Can you work these out from the model? Positions are in its coordinate system, mm. Give positions to 0.01 mm unless a question says otherwise; leave off trailing zeros. Order: outer loops, then holes, each group sorted by start corner. A loop starts at its lowest first (then second) coordinate and runs counter-clockwise, first axis right, second up. Notation, with made-up numbers: (7, -2.5) -> (28, -2.5) arc R24 cw to (28, 27.5) -> close; hole circle Ø10 at (28, 48). An arc over 180 degrees is marked (long way). Answer as a JSON object with one key per item and string values.
```python
from build123d import *

# Parameters (mm, degrees)
SKETCH1_R           = 2
SKETCH1_W           = 56
SKETCH1_H           = 56
BOSS_EXTRUDE1_DEPTH = 1
SKETCH3_W           = 56
SKETCH3_H           = 56
BOSS_EXTRUDE3_DEPTH = 1


with BuildPart() as part:
    # Sketch1 → Boss-Extrude1 (new body)
    with BuildSketch(Plane.XY):
        with BuildLine():
            Line((40, -13), (40, 13))
            ThreePointArc((40, 13), (38.828427125, 15.828427125), (36, 17))
            ThreePointArc((36, 17), (33.171572875, 18.171572875), (32, 21))
            Line((32, 21), (32, 32))
            Line((32, 32), (21, 32))
            ThreePointArc((21, 32), (18.171572875, 33.171572875), (17, 36))
            ThreePointArc((17, 36), (15.828427125, 38.828427125), (13, 40))
            Line((13, 40), (-13, 40))
            ThreePointArc((-13, 40), (-15.828427125, 38.828427125), (-17, 36))
            ThreePointArc((-17, 36), (-18.171572875, 33.171572875), (-21, 32))
            Line((-21, 32), (-32, 32))
            Line((-32, 32), (-32, 9))
            ThreePointArc((-32, 9), (-33.464466094, 5.464466094), (-37, 4))
            ThreePointArc((-37, 4), (-41, 0), (-37, -4))
            ThreePointArc((-37, -4), (-33.464466094, -5.464466094), (-32, -9))
            Line((-32, -9), (-32, -32))
            Line((-32, -32), (-9, -32))
            ThreePointArc((-9, -32), (-5.464466094, -33.464466094), (-4, -37))
            ThreePointArc((-4, -37), (0, -41), (4, -37))
            ThreePointArc((4, -37), (5.464466094, -33.464466094), (9, -32))
            Line((9, -32), (32, -32))
            Line((32, -32), (32, -21))
            ThreePointArc((32, -21), (33.171572875, -18.171572875), (36, -17))
            ThreePointArc((36, -17), (38.828427125, -15.828427125), (40, -13))
        make_face()
        with Locations((-37, 0)):
            Circle(SKETCH1_R, mode=Mode.SUBTRACT)
        with Locations((-13, 36)):
            Circle(SKETCH1_R, mode=Mode.SUBTRACT)
        with Locations((0, -37)):
            Circle(SKETCH1_R, mode=Mode.SUBTRACT)
        with Locations((36, -13)):
            Circle(SKETCH1_R, mode=Mode.SUBTRACT)
        with Locations((36, 13)):
            Circle(SKETCH1_R, mode=Mode.SUBTRACT)
        with Locations((13, 36)):
            Circle(SKETCH1_R, mode=Mode.SUBTRACT)
        Rectangle(SKETCH1_W, SKETCH1_H, mode=Mode.SUBTRACT)
    extrude(amount=BOSS_EXTRUDE1_DEPTH)

    # Sketch3 → Boss-Extrude3 (add)
    with BuildSketch(Plane.XY.offset(1)):
        Rectangle(SKETCH3_W, SKETCH3_H)
    extrude(amount=-BOSS_EXTRUDE3_DEPTH)


solid = part.part
```
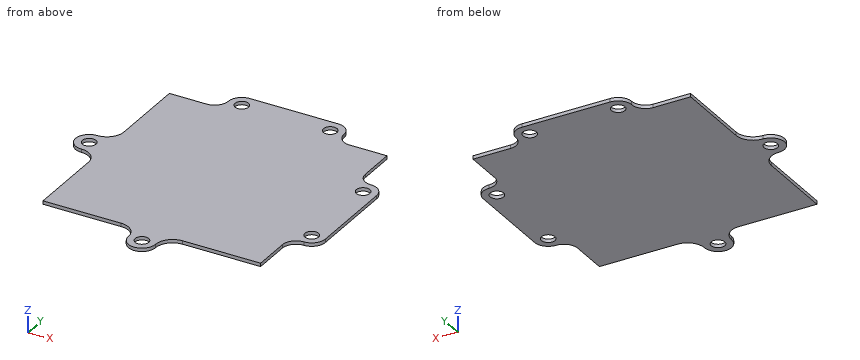
1. If we section it at A-A on x = 0: Please give me the cut outline in (y, z).
Worked answers:
{"outline": "(-41, 0) -> (-39, 0) -> (-39, 1) -> (-41, 1) -> close; (-35, 0) -> (40, 0) -> (40, 1) -> (-35, 1) -> close"}
2. If we section it at C-C on y = 12: Please give me the cut outline in (x, z), then the cut area to 3 significant figures.
Worked answers:
{"outline": "(-32, 0) -> (34.27, 0) -> (34.27, 1) -> (-32, 1) -> close; (37.73, 0) -> (40, 0) -> (40, 1) -> (37.73, 1) -> close", "area": "68.5 mm²"}
3. If we section it at D-D on x = 31: Please give me the cut outline in (y, z).
Worked answers:
{"outline": "(-32, 0) -> (32, 0) -> (32, 1) -> (-32, 1) -> close"}
4. Please list where these lines run through material, in increasing order: L1, parallel to Y at x = 36, z = 0.75; L2, parallel to Y at x = 13, z = 0.8; L3, parallel to Y at x = -37, z = 0.2.
Worked answers:
{"L1": "-17 to -15, -11 to 11, 15 to 17", "L2": "-32 to 34, 38 to 40", "L3": "-4 to -2, 2 to 4"}
5. Will these pins go through, and if not, where does the flat tip stop? pin 1 Ø0.5 at (x, z) = (-22, 0.5) entering from -Y; pin 2 Ø0.5 at (x, z) = (26.5, 0.5) entering from +Y; pin 3 Ø0.5 at (y, z) = (-25, 0.5) entering from +X; pin 4 Ø3.5 at (x, y) = (36, 13) entering from +Z.
Worked answers:
{"pin 1": "y = -32", "pin 2": "y = 32", "pin 3": "x = 32", "pin 4": "through"}
6. If we section it at B-B on z = 0.85: Count the separate pieces of the cut face and the enclosed holes in it, then the cut area to 3 significant figures.
Worked answers:
{"separate pieces": "1", "enclosed holes": "6", "area": "4,720 mm²"}
